Build history of the part. All positions in model axes, mm. Face numbers are marked on the shaded views. A direction names the side the tool comes from. Give positions to 0.01 mm unless a question says otherwise; leave off trailing zeros. Loops run counter-clockwise (first coordinate to the right, second up) from the corner with the lowest first, then second, coordinate; pieces in that order, holes last. Notation, with made-up numbers: (53.5, 18.5) - (103.5, 18.5) arc R31 ccw to (103.5, 44.5) - close; hole circle Ø4 at (-39.75, 5). An arc over 180 degrees is marked (long way). Return JSON: item names as keys, results as strings. Group by question number.
1) Drop flat-ended pins along their axis: pin 1 (1 mm diameter, centred on x = 28.91, z = 1.7, fed in from -Y); pin 2 (1 mm diameter, centred on x = 22.5, z = 3.5, fed in from -Y); pin 3 (1.9 mm diameter, centred on x = -28.87, z = 1.7, fed in from +Y); pin 4 (6 mm diameter, centred on x = 12, y = -2, fed in from +Z). Give the stop position or say it passes through.
2) Drill centre lines: probe 1 along Y at (x, z) = (0, 6.3); probe 2 along X at (y, z) = (7, 3.25); probe 3 along Z at (x, y) = (6.5, -15). Where is each one in solid material? Low to high. Write a range as from..to.
3) 3-axis set-ups, long thin cutter, end or side, ignore diameter. For the marked faces 1, 2 and 3: which of +Z, -Z, +X, -X, +Y, -Y reach the whole face in a straight line?
4) Mould opens along X. For the marked faces 4, 5 and 6 say: released by +X, released by -X, zero draft, split by the parting line, or undercut.
5) Slice it at A-A (x = 0). List the corners of the cut face in (y, z), and give its area (3 significant figures).
6) Slice it at B-B (y = 0). List the corners of the cut face in (x, z).
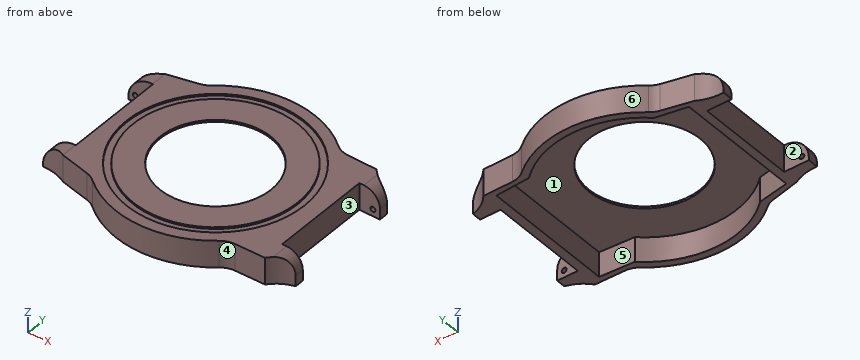
```python
from build123d import *

# Parameters (mm, degrees)
PAD_DEPTH       = 6.5
POCKET_DEPTH    = 6
SKETCH002_R     = 13.5
POCKET001_DEPTH = 1
SKETCH003_W     = 5.4
SKETCH003_H     = 6.5
PAD001_DEPTH    = 5
POCKET002_DEPTH = 10
SKETCH008_R     = 0.6
POCKET003_DEPTH = 2
SKETCH009_R     = 0.6
POCKET004_DEPTH = 2
FILLET_R        = 3.9
FILLET001_R     = 3.9
FILLET002_R     = 5
FILLET003_R     = 5
FILLET004_R     = 5
FILLET005_R     = 5
SKETCH010_W     = 3.95
SKETCH010_H     = 6.5
PAD002_DEPTH    = 6
POCKET005_DEPTH = 10
SKETCH012_R     = 0.6
POCKET006_DEPTH = 2
SKETCH013_R     = 0.6
POCKET007_DEPTH = 2
FILLET006_R     = 5.9
FILLET007_R     = 5.9
SKETCH014_R     = 21.6
SKETCH014_R_2   = 20
POCKET008_DEPTH = 0.4


with BuildPart() as part:
    # Sketch → Pad (new body)
    with BuildSketch(Plane.XY):
        with BuildLine():
            Line((-24.57081, 16), (-24.57081, -16))
            Line((-24.57081, -16), (-16.285883, -17.9))
            ThreePointArc((-16.285883, -17.9), (0.22069, -24.198994), (16.609636, -17.6))
            Line((16.609636, -17.6), (25.608386, -17.45))
            Line((25.608386, 17.45), (25.608386, -17.45))
            Line((16.609636, 17.6), (25.608386, 17.45))
            ThreePointArc((16.609636, 17.6), (0.22069, 24.198994), (-16.285883, 17.9))
            Line((-24.57081, 16), (-16.285883, 17.9))
        make_face()
    extrude(amount=PAD_DEPTH)

    # Sketch001 → Pocket (cut)
    with BuildSketch(Plane.XY):
        with BuildLine():
            Line((-15.242949, 16.55), (-22.620449, 15.2))
            Line((-22.620449, 15.2), (-22.620449, -15.2))
            Line((-22.620449, -15.2), (-15.242949, -16.55))
            ThreePointArc((-15.242949, -16.55), (0, -22.5), (15.242949, -16.55))
            Line((15.242949, -16.55), (23.527875, -16.05))
            Line((23.527875, 16.05), (23.527875, -16.05))
            Line((15.242949, 16.55), (23.527875, 16.05))
            ThreePointArc((15.242949, 16.55), (0, 22.5), (-15.242949, 16.55))
        make_face()
    extrude(amount=POCKET_DEPTH, mode=Mode.SUBTRACT)

    # Sketch002 (on Face19 of Pocket) → Pocket001 (cut)
    with BuildSketch(Plane(origin=(0, 0, 6), x_dir=(1, 0, 0), z_dir=(0, 0, -1))):
        Circle(SKETCH002_R)
    extrude(amount=-POCKET001_DEPTH, mode=Mode.SUBTRACT)

    # Sketch003 (on Face6 of Pocket001) → Pad001 (join)
    with BuildSketch(Plane.YZ.offset(25.608386)):
        with Locations((-14.75, 3.25)):
            Rectangle(SKETCH003_W, SKETCH003_H)
        with Locations((14.75, 3.25)):
            Rectangle(SKETCH003_W, SKETCH003_H)
    extrude(amount=PAD001_DEPTH)

    # Sketch006 → Pocket002 (cut)
    with BuildSketch(Plane.XY.offset(10)):
        with BuildLine():
            ThreePointArc((25.608386, 17.45), (27.842824, 15.439634), (30.608386, 14.262368))
            Line((30.608386, 17.45), (30.608386, 14.262368))
            Line((30.608386, 17.45), (25.608386, 17.45))
        make_face()
        with BuildLine():
            ThreePointArc((30.608386, -14.262368), (27.842824, -15.439634), (25.608386, -17.45))
            Line((30.608386, -17.45), (25.608386, -17.45))
            Line((30.608386, -14.262368), (30.608386, -17.45))
        make_face()
    extrude(amount=-POCKET002_DEPTH, mode=Mode.SUBTRACT)

    # Sketch008 (on Face27 of Pocket002) → Pocket003 (cut)
    with BuildSketch(Plane(origin=(0, -12.05, 0), x_dir=(-1, 0, 0), z_dir=(0, 1, 0))):
        with Locations((-28.908386, 1.7)):
            Circle(SKETCH008_R)
    extrude(amount=-POCKET003_DEPTH, mode=Mode.SUBTRACT)

    # Sketch009 (on Face26 of Pocket003) → Pocket004 (cut)
    with BuildSketch(Plane.XZ.offset(-12.05)):
        with Locations((28.908386, 1.7)):
            Circle(SKETCH009_R)
    extrude(amount=-POCKET004_DEPTH, mode=Mode.SUBTRACT)

    # Fillet
    fillet_edges = [part.edges().sort_by_distance(p)[0] for p in [
        (30.608386, -13.156184, 6.5),
    ]]
    fillet(fillet_edges, radius=FILLET_R)

    # Fillet001
    fillet001_edges = [part.edges().sort_by_distance(p)[0] for p in [
        (30.608386, 13.156184, 6.5),
    ]]
    fillet(fillet001_edges, radius=FILLET001_R)

    # Fillet002
    fillet002_edges = [part.edges().sort_by_distance(p)[0] for p in [
        (16.609636, -17.6, 3.25),
    ]]
    fillet(fillet002_edges, radius=FILLET002_R)

    # Fillet003
    fillet003_edges = [part.edges().sort_by_distance(p)[0] for p in [
        (16.609636, 17.6, 3.25),
    ]]
    fillet(fillet003_edges, radius=FILLET003_R)

    # Fillet004
    fillet004_edges = [part.edges().sort_by_distance(p)[0] for p in [
        (-16.285883, -17.9, 3.25),
    ]]
    fillet(fillet004_edges, radius=FILLET004_R)

    # Fillet005
    fillet005_edges = [part.edges().sort_by_distance(p)[0] for p in [
        (-16.285883, 17.9, 3.25),
    ]]
    fillet(fillet005_edges, radius=FILLET005_R)

    # Sketch010 (on Face4 of Fillet005) → Pad002 (join)
    with BuildSketch(Plane(origin=(-24.57081, 0, 0), x_dir=(0, -1, 0), z_dir=(-1, 0, 0))):
        with Locations((-14.025, 3.25)):
            Rectangle(SKETCH010_W, SKETCH010_H)
        with Locations((14.025, 3.25)):
            Rectangle(SKETCH010_W, SKETCH010_H)
    extrude(amount=PAD002_DEPTH)

    # Sketch011 (on Face6 of Pad002) → Pocket005 (cut)
    with BuildSketch(Plane.XY.offset(6.5)):
        with BuildLine():
            ThreePointArc((-30.57081, 14.6), (-27.470381, 14.869592), (-24.57081, 16))
            Line((-24.57081, 16), (-30.57081, 16))
            Line((-30.57081, 16), (-30.57081, 14.6))
        make_face()
        with BuildLine():
            ThreePointArc((-24.57081, -16), (-27.470381, -14.869592), (-30.57081, -14.6))
            Line((-30.57081, -14.6), (-30.57081, -16))
            Line((-30.57081, -16), (-24.57081, -16))
        make_face()
    extrude(amount=-POCKET005_DEPTH, mode=Mode.SUBTRACT)

    # Sketch012 (on Face23 of Pocket005) → Pocket006 (cut)
    with BuildSketch(Plane(origin=(0, -12.05, 0), x_dir=(-1, 0, 0), z_dir=(0, 1, 0))):
        with Locations((28.87081, 1.7)):
            Circle(SKETCH012_R)
    extrude(amount=-POCKET006_DEPTH, mode=Mode.SUBTRACT)

    # Sketch013 (on Face21 of Pocket006) → Pocket007 (cut)
    with BuildSketch(Plane.XZ.offset(-12.05)):
        with Locations((-28.87081, 1.7)):
            Circle(SKETCH013_R)
    extrude(amount=-POCKET007_DEPTH, mode=Mode.SUBTRACT)

    # Fillet006
    fillet006_edges = [part.edges().sort_by_distance(p)[0] for p in [
        (-30.57081, 13.325, 6.5),
    ]]
    fillet(fillet006_edges, radius=FILLET006_R)

    # Fillet007
    fillet007_edges = [part.edges().sort_by_distance(p)[0] for p in [
        (-30.57081, -13.325, 6.5),
    ]]
    fillet(fillet007_edges, radius=FILLET007_R)

    # Sketch014 (on Face4 of Fillet007) → Pocket008 (cut)
    with BuildSketch(Plane.XY.offset(6.5)):
        Circle(SKETCH014_R)
        Circle(SKETCH014_R_2, mode=Mode.SUBTRACT)
    extrude(amount=-POCKET008_DEPTH, mode=Mode.SUBTRACT)


solid = part.part
```
Results:
{
 "1": {"pin 1": "y = -15.11", "pin 2": "y = -17.51", "pin 3": "y = 14.77", "pin 4": "z = 6.5"},
 "2": {"probe 1": "-24.2..-21.6, -20..-13.5, 13.5..20, 21.6..24.2", "probe 2": "-24.57..-22.62, 23.53..25.61", "probe 3": "6..6.5"},
 "3": {"face 1": "-Z", "face 2": "+Z, -Z, -X", "face 3": "+Z, -Z, +X"},
 "4": {"face 4": "released by +X", "face 5": "undercut", "face 6": "split by the parting line"},
 "5": {"outline": "(-24.2, 0) - (-22.5, 0) - (-22.5, 6) - (-13.5, 6) - (-13.5, 6.5) - (-20, 6.5) - (-20, 6.1) - (-21.6, 6.1) - (-21.6, 6.5) - (-24.2, 6.5) - close; (13.5, 6) - (22.5, 6) - (22.5, 0) - (24.2, 0) - (24.2, 6.5) - (21.6, 6.5) - (21.6, 6.1) - (20, 6.1) - (20, 6.5) - (13.5, 6.5) - close", "area": "29.8 mm2"},
 "6": {"outline": "(-24.57, 0) - (-22.62, 0) - (-22.62, 6) - (-13.5, 6) - (-13.5, 6.5) - (-20, 6.5) - (-20, 6.1) - (-21.6, 6.1) - (-21.6, 6.5) - (-24.57, 6.5) - close; (13.5, 6) - (23.53, 6) - (23.53, 0) - (25.61, 0) - (25.61, 6.5) - (21.6, 6.5) - (21.6, 6.1) - (20, 6.1) - (20, 6.5) - (13.5, 6.5) - close"}
}
